Design review of the part built by this model. Coordinates are the model's own, in mm. Face numbers are marked on the shaded views. A direction names the side the tool comes from. Coordinates: 2 decimals unless noted, no trailing zeros. Loops run counter-clockwise (first coordinate to the right, second up) from the corner with the lowest first, then second, coordinate; pieces in that order, holes last.
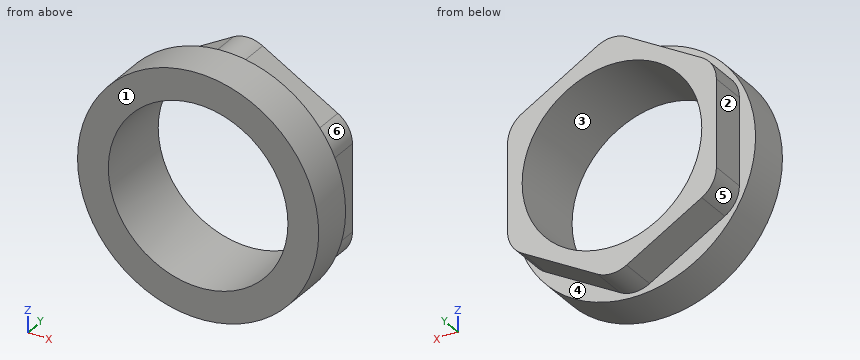
Autodesk Inventor part; units mm, degrees
ref_plane "YZ Plane" through (0, 0, 0) normal (1, 0, 0) x (0, 1, 0)
ref_plane "XZ Plane" through (0, 0, 0) normal (0, 1, 0) x (-1, 0, 0)
ref_plane "XY Plane" through (0, 0, 0) normal (0, 0, 1) x (1, 0, 0)
sketch "Sketch1" plane through (0, 0, 0) normal (0, 1, 0) x (-1, 0, 0)
  circle A0 centre (0, 0) radius 9.2
  circle A1 centre (0, 0) radius 12.35
  dimension "d0" = 18.4
  dimension "d1" = 3.15
  dimension "d9" = 24.7
extrude "Extrusion1" add sketch "Sketch1" along normal blind 4.45
thread "Thread1"
sketch "Sketch2" plane through (0, 4.45, 0) normal (0, 1, 0) x (1, 0, 0)
  line L0 (-10.6954, 6.175) -> (0, 12.35)
  line L1 (0, 12.35) -> (10.6954, 6.175)
  line L2 (10.6954, 6.175) -> (10.6954, -6.175)
  line L3 (10.6954, -6.175) -> (0, -12.35)
  line L4 (0, -12.35) -> (-10.6954, -6.175)
  line L5 (-10.6954, -6.175) -> (-10.6954, 6.175)
  circle A0 centre (0, 0) radius 9.2
extrude "Extrusion2" add sketch "Sketch2" along normal blind 3.81
fillet "Fillet1" radius 3 6 edges at (10.6954, 6.355, 6.175) (10.6954, 6.355, -6.175) (0, 6.355, -12.35) (-10.6954, 6.355, -6.175) (-10.6954, 6.355, 6.175) (0, 6.355, 12.35)
properties part number "gearProx"
Q1. Take a section at B-B, the plane z = 9.5. Write out the cut boundary in (x, y), then the cut area to 3 significant figures.
Q2. Clearance check with flat-ended pins moving along their axes: pin 1 Ø1.1 at (y, z) = (6, 2) entering from +X; pin 2 Ø1 at (x, y) = (1.5, 7) entering from +Z; pin 3 Ø2 at (x, y) = (8.5, 5) entering from -Z; pin 4 Ø11 at (x, z) = (0, 0) entering from +Y. State where each tip first meets the part, or that it passes through.
Q3. For line 1 (X direction, y = 6.25, z = 0); line 2 (Z direction, x = 0, y = 2); line 3 (Z direction, x = 0, y = 6.5), list the stretches that pass through material, from the lowest coordinate up.
Q4. The part is to be moulded in two halves that separate along X. For the marked faces 1, 2 and 3, say which applies: pulls with the +X half, pulls with the -X half, needs draft (parallel to the pull), parting line crosses it, or undercut.
Q5. Machinability: for the marked faces 4, 5 and 6, which of the approach directions +Z, -Z, +X, -X, +Y, -Y give a long, thin tool a straight path to every point of the face, cutting with its end or side? Answer none if there is none.
Q6. Take a section at A-A, the plane y = 7.5. Write out the cut boundary in (x, z), then the cut area to 3 significant figures.
Entries:
1. outline: (-7.89, 0) - (7.89, 0) - (7.89, 4.45) - (4.94, 4.45) - (4.94, 8.26) - (-4.94, 8.26) - (-4.94, 4.45) - (-7.89, 4.45) - close
1. area: 108 mm2
2. pin 1: stops at x = 10.7
2. pin 2: stops at z = 11.71
2. pin 3: stops at z = -9.68
2. pin 4: passes through
3. line 1: x = -10.7 to -9.2, 9.2 to 10.7
3. line 2: z = -12.35 to -9.2, 9.2 to 12.35
3. line 3: z = -11.89 to -9.2, 9.2 to 11.89
4. face 1: needs draft
4. face 2: pulls with the -X half
4. face 3: undercut
5. face 4: +Y
5. face 5: -Z, -X, +Y
5. face 6: +Z, +X, +Y
6. outline: (-10.7, -4.44) arc R3 ccw to (-9.2, -7.04) - (-1.5, -11.48) arc R3 ccw to (1.5, -11.48) - (9.2, -7.04) arc R3 ccw to (10.7, -4.44) - (10.7, 4.44) arc R3 ccw to (9.2, 7.04) - (1.5, 11.48) arc R3 ccw to (-1.5, 11.48) - (-9.2, 7.04) arc R3 ccw to (-10.7, 4.44) - close; hole circle Ø18.4 at (0, 0)
6. area: 127 mm2
